from build123d import *

# Parameters (mm, degrees)
F1_DEPTH = 99.06
F2_SIZE  = 1.27


with BuildPart() as f1:
    # F0 (on Top) → F1 (new body)
    with BuildSketch(Plane.XY):
        Polygon((-3.223582, 1.106647), (-1.687731, -1.672163), (1.486715, -1.731482), (3.125309, 0.988009), (1.589458, 3.766819), (-1.584988, 3.826138), align=None)
    extrude(amount=F1_DEPTH)

    # F2
    f2_edges = [f1.edges().sort_by_distance(p)[0] for p in [
        (-2.404285, 2.466393, 0),
        (-2.455657, -0.282758, 0),
        (-0.100508, -1.701823, 0),
        (2.306012, -0.371737, 0),
        (2.357384, 2.377414, 0),
        (0.002235, 3.796479, 0),
        (-2.404285, 2.466393, 99.06),
        (-2.455657, -0.282758, 99.06),
        (-0.100508, -1.701823, 99.06),
        (2.306012, -0.371737, 99.06),
        (2.357384, 2.377414, 99.06),
        (0.002235, 3.796479, 99.06),
    ]]
    chamfer(f2_edges, length=F2_SIZE)


solid = f1.part
Source: CAD feature listing. Evaluate the final solid. Frame: model axes, mm. Round coordinates to 2 decimals unless told otherwise and drop trailing zeros. Loops run counter-clockwise (first coordinate to the right, second up) from the corner with the lowest first, then second, coordinate; pieces in that order, holes last. Notation, with made-up numbers: (87.25, -17.75) - (126.25, -17.75) arc R34 ccw to (126.25, 13.25) - close; hole circle Ø9 at (-17, 36). An arc over 180 degrees is marked (long way). Write item = value, one per line. Start each with the question number.
(1) Ray query, line 1 along Y through (x, z) = (-1.5, 7.5); line 2 along Y through (x, z) = (-3, 76); line 3 along X through (y, z) = (1.2, 60.5). Return the intervals inside material, ascending. Write a range as from..to.
(2) Section query A-A, the plane z = 45. Output: boundary loops of the cut face in (x, y), plus the area to 3 significant figures.
(3) Pin query (flat end, axial travel): pin 1 (1.5 mm diameter, centred on x = 2, y = 3, fed in from +Z); pin 2 (1 mm diameter, centred on x = 2, y = 3, fed in from +Z); pin 3 (1 mm diameter, centred on x = -2.5, y = 3, fed in from +Z). Return the tip coordinate at first contact, or that it passes through.
Conclusion:
q1.line_1 = -1.68..3.82
q1.line_2 = 0.7..1.48
q1.line_3 = -3.17..3.01
q2.outline = (-3.22, 1.11) - (-1.69, -1.67) - (1.49, -1.73) - (3.13, 0.99) - (1.59, 3.77) - (-1.58, 3.83) - close
q2.area = 26.2 mm2
q3.pin_1 = 98.55
q3.pin_2 = 98.3
q3.pin_3 = 97.93
